```python
from build123d import *

# Parameters (mm, degrees)
F1_DEPTH = 1270
F2_DEPTH = 127
F3_DEPTH = 25.4


with BuildPart() as f1:
    # F0 (on Front) → F1 (new body)
    with BuildSketch(Plane.XZ):
        Polygon((127, 0), (0, 0), (0, -254), (406.4, -254), (406.4, 0), (279.4, 0), (279.4, 256.7683129114), (656.6807052125, -254), (1033.9614104249, 256.7683129114), (1033.9614104249, 0), (906.9614104249, 0), (906.9614104249, -254), (1313.3614104249, -254), (1313.3614104249, 0), (1186.3614104249, 0), (1186.3614104249, 381), (1313.3614104249, 381), (1313.3614104249, 635), (1110.1614104249, 635), (656.6807052125, 190.5), (203.2, 635), (0, 635), (0, 381), (127, 381), align=None)
    extrude(amount=F1_DEPTH)

    # F2 (add): a face of the model
    f2_faces = [f1.faces().sort_by_distance(p)[0] for p in [
        (656.6807052125, 0, 153.5673559102),
    ]]
    extrude(f2_faces, amount=-F2_DEPTH)

    # F0 (on Front) → F3 (join)
    with BuildSketch(Plane.XZ):
        Polygon((127, 0), (0, 0), (0, -254), (406.4, -254), (406.4, 0), (279.4, 0), (279.4, 256.7683129114), (656.6807052125, -254), (1033.9614104249, 256.7683129114), (1033.9614104249, 0), (906.9614104249, 0), (906.9614104249, -254), (1313.3614104249, -254), (1313.3614104249, 0), (1186.3614104249, 0), (1186.3614104249, 381), (1313.3614104249, 381), (1313.3614104249, 635), (1110.1614104249, 635), (656.6807052125, 190.5), (203.2, 635), (0, 635), (0, 381), (127, 381), align=None)
    extrude(amount=F3_DEPTH)


solid = f1.part
```
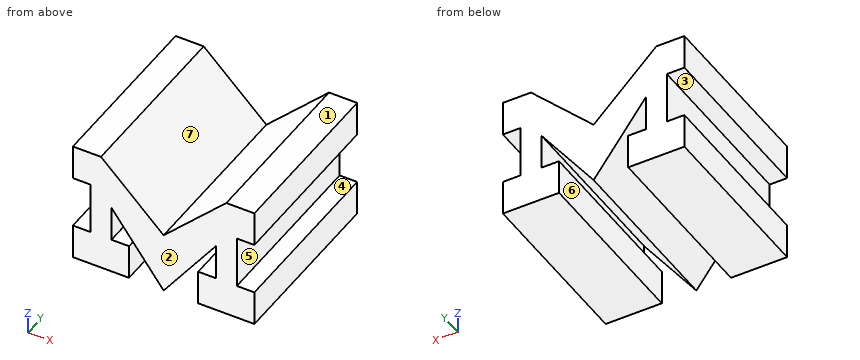
Can you work these out from the model? Positions are in its coordinate system, mm. Face numbers are marked on the shaded views. A direction names the side the tool comes from. Give positions to 0.01 mm unless a question says otherwise; leave off trailing zeros. Loops run counter-clockwise (first coordinate to the right, second up) from the corner with the lowest first, then second, coordinate; pieces in that order, holes last. Notation, with made-up numbers: M 71,68.25 L 91,68.25 A23 cw 91,89.25 Z; hole C 89.5,47.5 d8. An arc over 180 degrees is marked long. Use one line per item in the form item = value. Start each with the question number.
(1) I'm going to push flat-ended pins straight in: P1, Ø5, axis at x = 728.5, y = -952, coming from the -Z side; P2, Ø5, axis at x = 475.5, y = -310.5, coming from the -Z side; P3, Ø12, axis at y = -566, z = 287.5, coming from the +X side. Where does each tip first touch, or does it pass through?
(2) Thinking about a two-plate mould opening in Z: for the marked faces 1, 2, 3 and 4, which applies, released by +Z, released by -Z, zero draft, split by the parting line, or undercut?
(3) I want a section at B-B, the plane x = 991. Write out the boundary of the cut face in (y, z).
(4) I want a section at C-C, the plane y = -1029. Write out the boundary of the cut face in (x, z), and give its area (3 significant figures).
(5) On a 3-axis mill with a long thin cutter (end or side, diameter ignored), from which of +Z, -Z, +X, -X, +Y, -Y can I reach the whole of each face in a straight line? I mean the marked faces 5, 6 and 7. Say none if no direction works.
(6) I want a section at D-D, the plane z = -41. Write out the boundary of the cut face in (x, y), and give its area (3 significant figures).
(7) Please list where these lines run through material, in increasing order: line 1 (Z direction, x = 122.5, y = -133); line 2 (X direction, y = -113.5, z = -30.5); line 3 (X direction, y = -840, z = -100.5).
(8) I want a section at A-A, the plane z = 500.5. Write out the boundary of the cut face in (x, y).
Worked out:
q1.P1 = -160.15
q1.P2 = -12.1
q1.P3 = 1186.36
q2.face_1 = released by +Z
q2.face_2 = zero draft
q2.face_3 = undercut
q2.face_4 = undercut
q3.outline = M -1270,-254 L 0,-254 L 0,0 L -1270,0 Z; M -1270,198.61 L 0,198.61 L 0,518.2 L -1270,518.2 Z
q4.outline = M 0,-254 L 406.4,-254 L 406.4,0 L 279.4,0 L 279.4,256.77 L 656.68,-254 L 1033.96,256.77 L 1033.96,0 L 906.96,0 L 906.96,-254 L 1313.36,-254 L 1313.36,0 L 1186.36,0 L 1186.36,381 L 1313.36,381 L 1313.36,635 L 1110.16,635 L 656.68,190.5 L 203.2,635 L 0,635 L 0,381 L 127,381 L 127,0 L 0,0 Z
q4.area = 741,000 mm²
q5.face_5 = +X, +Y, -Y
q5.face_6 = -Z, +Y, -Y
q5.face_7 = +Z, +Y, -Y
q6.outline = M 0,-1270 L 406.4,-1270 L 406.4,0 L 0,0 Z; M 499.35,-1270 L 814.01,-1270 L 814.01,0 L 499.35,0 Z; M 906.96,-1270 L 1313.36,-1270 L 1313.36,0 L 906.96,0 Z
q6.area = 1,430,000 mm²
q7.line_1 = -254 to 0, 381 to 635
q7.line_2 = 0 to 406.4, 491.59 to 821.77, 906.96 to 1313.36
q7.line_3 = 0 to 406.4, 543.3 to 770.06, 906.96 to 1313.36
q8.outline = M 0,-1270 L 340.42,-1270 L 340.42,0 L 0,0 Z; M 972.94,-1270 L 1313.36,-1270 L 1313.36,0 L 972.94,0 Z
